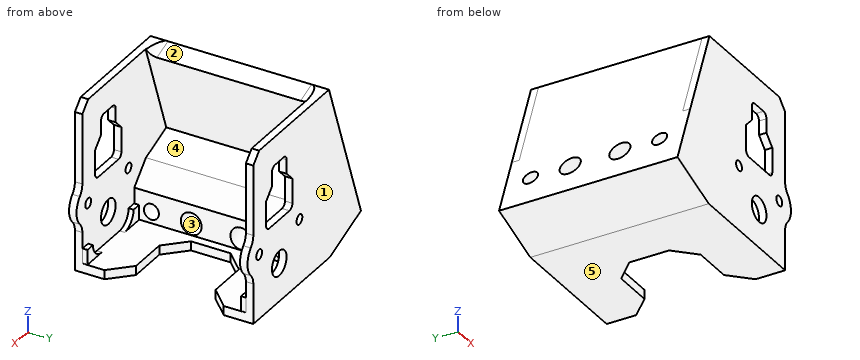
from build123d import *

# Parameters (mm, degrees)
SKETCH1_W                  = 17.8
SKETCH1_H                  = 30
SKETCH1_R                  = 1
SKETCH1_R_2                = 2.5
BOSS_EXTRUDE1_DEPTH        = 1.5
SKETCH2_W                  = 9
SKETCH2_H                  = 6
SKETCH2_W_2                = 5
SKETCH2_H_2                = 5.830943002
CUT_EXTRUDE1_DEPTH         = 20.247337478
CHAMFER1_SIZE              = 2
FILLET1_R                  = 1
BOSS_EXTRUDE2_DEPTH        = 1
SKETCH4_W                  = 12
SKETCH4_H                  = 17.95
BOSS_EXTRUDE3_DEPTH        = 4
BOSS_EXTRUDE4_DEPTH        = 35.9
SKETCH6_W                  = 12.770133269
SKETCH6_H                  = 35.9
BOSS_EXTRUDE5_DEPTH        = 11.41
F_3_0_MM_DOWEL_HOLES1_D    = 3
F_4_2_4_2_DIAMETER_HOLE1_D = 4.2
SKETCH12_W                 = 17.8
SKETCH12_H                 = 1.5
BOSS_EXTRUDE6_DEPTH        = 4
CHAMFER2_SIZE              = 2
SKETCH13_W                 = 26.167642811
SKETCH13_H                 = 35.9
BOSS_EXTRUDE7_DEPTH        = 1.840000002
CHAMFER3_SIZE              = 4
CHAMFER4_SIZE              = 4
SKETCH14_W                 = 16
SKETCH14_H                 = 8
CUT_EXTRUDE2_DEPTH         = 56.735892419
CHAMFER5_SIZE              = 4
BOSS_EXTRUDE8_DEPTH        = 1.5
BOSS_EXTRUDE9_START        = -34.4
BOSS_EXTRUDE9_DEPTH        = 1.5
FILLET2_R                  = 3
BOSS_EXTRUDE10_START       = -1.5
BOSS_EXTRUDE10_DEPTH       = 1.5
BOSS_EXTRUDE11_START       = -35.9
BOSS_EXTRUDE11_DEPTH       = 1.5
SKETCH18_W                 = 19.259010622
SKETCH18_H                 = 32.9
BOSS_EXTRUDE12_DEPTH       = 4
FILLET3_R                  = 2


# Some blends are built 0.0001 mm under size
with BuildPart() as part:
    # Sketch1 → Boss-Extrude1 (new body)
    with BuildSketch(Plane(origin=(0, 0, 0), x_dir=(1, 0, 0), z_dir=(0, 1, 0))):
        with Locations((0, -2)):
            Rectangle(SKETCH1_W, SKETCH1_H)
        with Locations(Location((-6.9, 0, 0), (0, 0, 270))):
            Circle(SKETCH1_R, mode=Mode.SUBTRACT)
        with Locations(Location((6.9, 0, 0), (0, 0, 270))):
            Circle(SKETCH1_R, mode=Mode.SUBTRACT)
        with Locations(Location((0, 5.3, 0), (0, 0, 270))):
            Circle(SKETCH1_R_2, mode=Mode.SUBTRACT)
    extrude(amount=BOSS_EXTRUDE1_DEPTH)

    # Sketch2 → Cut-Extrude1 (cut, through all)
    with BuildSketch(Plane(origin=(0, 1.5, 0), x_dir=(1, 0, 0), z_dir=(0, 1, 0))):
        with Locations((0, -6.5)):
            Rectangle(SKETCH2_W, SKETCH2_H)
        with Locations((0, -12.415471501)):
            Rectangle(SKETCH2_W_2, SKETCH2_H_2)
    extrude(amount=-CUT_EXTRUDE1_DEPTH, mode=Mode.SUBTRACT)

    # Chamfer1
    chamfer1_edges = [part.edges().sort_by_distance(p)[0] for p in [
        (2.5, 0.75, 9.5),
        (-2.5, 0.75, 9.5),
    ]]
    chamfer(chamfer1_edges, length=CHAMFER1_SIZE - 0.0001)  # a hair under: the kernel refuses the full size

    # Fillet1
    fillet1_edges = [part.edges().sort_by_distance(p)[0] for p in [
        (4.5, 0.75, 3.5),
        (2.5, 0.75, 15.330943002),
        (-2.5, 0.75, 15.330943002),
        (-4.5, 0.75, 3.5),
    ]]
    fillet(fillet1_edges, radius=FILLET1_R)

    # Sketch3 → Boss-Extrude2 (add)
    with BuildSketch(Plane(origin=(0, 1.5, 0), x_dir=(1, 0, 0), z_dir=(0, 1, 0))):
        with BuildLine():
            Line((8.84, 8.16), (6.959390471, 8.16))
            ThreePointArc((6.959390471, 8.16), (6.042112051, 10.284532913), (3.900010938, 11.159999998))
            Line((3.900010938, 11.159999998), (-3.900010938, 11.159999998))
            ThreePointArc((-3.900010938, 11.159999998), (-6.04211205, 10.284532912), (-6.959390471, 8.16))
            Line((-6.959390471, 8.16), (-8.84, 8.16))
            Line((-8.84, 8.16), (-8.84, 12.94))
            Line((-8.84, 12.94), (8.84, 12.94))
            Line((8.84, 12.94), (8.84, 8.16))
        make_face()
    extrude(amount=BOSS_EXTRUDE2_DEPTH)

    # Sketch4 → Boss-Extrude3 (add)
    with BuildSketch(Plane.ZY.offset(8.9)):
        with Locations((-7, 8.975)):
            Rectangle(SKETCH4_W, SKETCH4_H)
    extrude(amount=BOSS_EXTRUDE3_DEPTH)

    # Mirror2: part across plane


with BuildPart() as part_1:
    add(part.part)
    add(part.part.mirror(Plane.ZX.offset(17.95)))

    # Sketch5 → Boss-Extrude4 (add)
    with BuildSketch(Plane(origin=(0, 35.9, 0), x_dir=(1, 0, 0), z_dir=(0, 1, 0))):
        Polygon((-12.9, 1), (-17.267642811, 13), (-12.9, 13), align=None)
    extrude(amount=-BOSS_EXTRUDE4_DEPTH)

    # Sketch6 → Boss-Extrude5 (add)
    with BuildSketch(Plane(origin=(-11.069592853, 0, 4.029002304), x_dir=(0.3420201433256634, 0, 0.9396926207859103), z_dir=(-0.9396926207859103, 0, 0.3420201433256634))):
        with Locations((-11.736819105, 17.95)):
            Rectangle(SKETCH6_W, SKETCH6_H)
    extrude(amount=BOSS_EXTRUDE5_DEPTH)

    # Ø3.0 mm Dowel Holes1 (through all)
    with Locations(Plane(origin=(-23.72675034, 0, 2.614356121), x_dir=(-0.34202014332566333, 0, -0.9396926207859103), z_dir=(-0.9396926207859104, 0, 0.3420201433256634))):
        with Locations((5.693417073, -4.95), (5.693417073, -30.95)):
            Hole(F_3_0_MM_DOWEL_HOLES1_D / 2)

    # Ø4.2 (4.2) Diameter Hole1 (through all)
    with Locations(Plane(origin=(-21.791485656, 0, 7.931452139), x_dir=(0.34202014332566333, 0, 0.9396926207859103), z_dir=(-0.9396926207859104, 0, 0.3420201433256634))):
        with Locations((-11.35175247, 12.95), (-11.35175247, 22.95)):
            Hole(F_4_2_4_2_DIAMETER_HOLE1_D / 2)

    # Sketch12 → Boss-Extrude6 (add)
    with BuildSketch(Plane.XY.offset(17)):
        with Locations((0, 35.15)):
            Rectangle(SKETCH12_W, SKETCH12_H)
        with Locations((0, 0.75)):
            Rectangle(SKETCH12_W, SKETCH12_H)
    extrude(amount=BOSS_EXTRUDE6_DEPTH)

    # Chamfer2
    chamfer2_edges = [part_1.edges().sort_by_distance(p)[0] for p in [
        (8.9, 35.15, 21),
        (-8.9, 35.15, 21),
        (-8.9, 0.75, 21),
        (8.9, 0.75, 21),
    ]]
    chamfer(chamfer2_edges, length=CHAMFER2_SIZE)

    # Sketch13 → Boss-Extrude7 (add)
    with BuildSketch(Plane(origin=(0, 0, -13), x_dir=(-1, 0, 0), z_dir=(0, 0, -1))):
        with Locations((4.183821406, 17.95)):
            Rectangle(SKETCH13_W, SKETCH13_H)
    extrude(amount=-BOSS_EXTRUDE7_DEPTH)

    # Chamfer3
    # the kernel refuses this chamfer: 4 mm, written as the material it adds along each edge
    with BuildSketch(Plane(origin=(-8.9, 0, -1), x_dir=(-0.9996219169112968, 0, -0.027495876610586216), z_dir=(0, 1, 0)), Plane(origin=(-8.9, 35.9, -1), x_dir=(0.027495876610586924, 0, 0.9996219169112968), z_dir=(0, -1, 0))) as chamfer3_piece_1:
        Polygon((CHAMFER3_SIZE * 0.999621916911, CHAMFER3_SIZE * 0.0274958766106), (-CHAMFER3_SIZE * 0.0274958766106, CHAMFER3_SIZE * 0.999621916911), (0, 0), align=None)
    extrude(amount=1.5)

    # Chamfer4
    chamfer4_edges = [part_1.edges().sort_by_distance(p)[0] for p in [
        (-8.9, 17.95, -1),
    ]]
    chamfer(chamfer4_edges, length=CHAMFER4_SIZE - 0.0001)  # a hair under: the kernel refuses the full size

    # Sketch14 → Cut-Extrude2 (cut, through all)
    with BuildSketch(Plane.XY.offset(-11.159999998)):
        with Locations((0.9, 21.95)):
            Rectangle(SKETCH14_W, SKETCH14_H)
        with Locations((0.9, 13.95)):
            Rectangle(SKETCH14_W, SKETCH14_H)
    extrude(amount=-CUT_EXTRUDE2_DEPTH, mode=Mode.SUBTRACT)

    # Chamfer5
    chamfer5_edges = [part_1.edges().sort_by_distance(p)[0] for p in [
        (-7.1, 9.95, -12.079999999),
        (-7.1, 25.95, -12.079999999),
        (8.9, 25.95, -12.079999999),
        (8.9, 9.95, -12.079999999),
    ]]
    chamfer(chamfer5_edges, length=CHAMFER5_SIZE)

    # Sketch15 → Boss-Extrude8 (add)
    with BuildSketch(Plane.XZ):
        with BuildLine():
            Line((8.9, 3.464101615), (8.9, -3.464101615))
            ThreePointArc((8.9, -3.464101615), (10.9, 0), (8.9, 3.464101615))
        make_face()
    extrude(amount=-BOSS_EXTRUDE8_DEPTH)

    # Sketch15<2> → Boss-Extrude9 (add)
    with BuildSketch(Plane.XZ.offset(BOSS_EXTRUDE9_START)):
        with BuildLine():
            Line((8.9, 3.464101615), (8.9, -3.464101615))
            ThreePointArc((8.9, -3.464101615), (10.9, 0), (8.9, 3.464101615))
        make_face()
    extrude(amount=-BOSS_EXTRUDE9_DEPTH)

    # Fillet2
    fillet2_edges = [part_1.edges().sort_by_distance(p)[0] for p in [
        (-12.9, 0.75, -1),
        (-12.9, 35.15, -1),
        (-8.9, 0.75, 3),
        (-8.9, 35.15, 3),
        (8.9, 0.75, -3.464101615),
        (8.9, 0.75, 3.464101615),
        (8.9, 35.15, 3.464101615),
        (8.9, 35.15, -3.464101615),
    ]]
    fillet(fillet2_edges, radius=FILLET2_R)

    # Sketch16 → Boss-Extrude10 (add)
    with BuildSketch(Plane(origin=(0, 35.9, 0), x_dir=(1, 0, 0), z_dir=(0, 1, 0)).offset(BOSS_EXTRUDE10_START)):
        with BuildLine():
            Line((-8.9, -4.242640687), (-8.9, -19))
            Line((-8.9, -19), (-6.9, -21))
            Line((-6.9, -21), (-17.03492323, -21))
            Line((-17.03492323, -21), (-23.621892803, -2.902449835))
            Line((-23.621892803, -2.902449835), (-14.695950669, 0.346327414))
            ThreePointArc((-14.695950669, 0.346327414), (-13.020571397, 0.456137573), (-11.548569895, -0.351430105))
            Line((-11.548569895, -0.351430105), (-9.778679656, -2.121320344))
            ThreePointArc((-9.778679656, -2.121320344), (-9.128361402, -3.09459039), (-8.9, -4.242640687))
        make_face()
    extrude(amount=BOSS_EXTRUDE10_DEPTH)

    # Sketch16<2> → Boss-Extrude11 (add)
    with BuildSketch(Plane(origin=(0, 35.9, 0), x_dir=(1, 0, 0), z_dir=(0, 1, 0)).offset(BOSS_EXTRUDE11_START)):
        with BuildLine():
            Line((-8.9, -4.242640687), (-8.9, -19))
            Line((-8.9, -19), (-6.9, -21))
            Line((-6.9, -21), (-17.03492323, -21))
            Line((-17.03492323, -21), (-23.621892803, -2.902449835))
            Line((-23.621892803, -2.902449835), (-14.695950669, 0.346327414))
            ThreePointArc((-14.695950669, 0.346327414), (-13.020571397, 0.456137573), (-11.548569895, -0.351430105))
            Line((-11.548569895, -0.351430105), (-9.778679656, -2.121320344))
            ThreePointArc((-9.778679656, -2.121320344), (-9.128361402, -3.09459039), (-8.9, -4.242640687))
        make_face()
    extrude(amount=BOSS_EXTRUDE11_DEPTH)

    # Sketch18 → Boss-Extrude12 (add)
    with BuildSketch(Plane(origin=(-21.791485656, 0, 7.931452139), x_dir=(0.34202014332566333, 0, 0.9396926207859103), z_dir=(-0.9396926207859104, 0, 0.3420201433256634))):
        with Locations((4.277752841, 17.95)):
            Rectangle(SKETCH18_W, SKETCH18_H)
    extrude(amount=-BOSS_EXTRUDE12_DEPTH)

    # Fillet3
    # the kernel refuses this fillet: 2 mm, written as the material it adds along each edge
    with BuildSketch(Plane(origin=(-21.733386334, 34.4, 22.710100717), x_dir=(0.3420201433256634, 0, 0.9396926207859104), z_dir=(0.9396926207859104, 0, -0.3420201433256634))) as fillet3_piece_1_section:
        with BuildLine():
            CenterArc((FILLET3_R, FILLET3_R), FILLET3_R, 180, 90)
            Line((0, FILLET3_R), (0, 0))
            Line((0, 0), (FILLET3_R, 0))
        make_face()
    fillet3_piece_1 = extrude(amount=9, mode=Mode.PRIVATE)
    fillet3_piece_1 = split(fillet3_piece_1, bisect_by=Plane(origin=(-14.648893953, 33.872369462, 21), z_dir=(0, 0, -1)), keep=Keep.TOP, mode=Mode.PRIVATE)
    add(fillet3_piece_1)
    with BuildSketch(Plane(origin=(-21.733386334, 1.5, 22.710100717), x_dir=(0, 1, 0), z_dir=(0.9396926207859104, 0, -0.3420201433256634))) as fillet3_piece_2_section:
        with BuildLine():
            CenterArc((FILLET3_R, FILLET3_R), FILLET3_R, 180, 90)
            Line((0, FILLET3_R), (0, 0))
            Line((0, 0), (FILLET3_R, 0))
        make_face()
    fillet3_piece_2 = extrude(amount=9, mode=Mode.PRIVATE)
    fillet3_piece_2 = split(fillet3_piece_2, bisect_by=Plane(origin=(-14.648893954, 2.027630538, 21), z_dir=(0, 0, -1)), keep=Keep.TOP, mode=Mode.PRIVATE)
    add(fillet3_piece_2)


solid = part_1.part
Geometry check sheet. Reference: the model listing, model coordinates, mm. Face numbers are marked on the shaded views. A direction names the side the tool comes from. Give positions to 0.01 mm unless a question says otherwise; leave off trailing zeros.
1. Scan lines: line 1 (Y direction, x = -11, z = -1); line 2 (X direction, y = 34.95, z = 0); line 3 (Z direction, x = -1.5, y = 33.5). Record each from-to range of solid material in increasing order.
Completed:
line 1: y = 0 to 1.5, 34.4 to 35.9
line 2: x = -24.68 to -7.9, -5.9 to 5.9, 7.9 to 10.9
line 3: z = -13 to -11.16
2. Depth check by flat-ended pin: pin 1 (12 mm diameter, centred on y = 9.5, z = -2.5, fed in from -X); pin 2 (2 mm diameter, centred on x = -7, y = 4, fed in from +Z); pin 3 (6 mm diameter, centred on x = -18, y = 27.5, fed in from +Z). Enter the tip coordinate at first touch or a pass-through.
Completed:
pin 1: stops at x = -27.77
pin 2: stops at z = -11.16
pin 3: stops at z = 21
3. Draft check along Z on the marked faces 1, 2 and 3. Enter one of: pulls with the +Z half, pulls with the -Z half, needs draft (parallel to the pull), parting line crosses it, or undercut.
Completed:
face 1: needs draft
face 2: pulls with the +Z half
face 3: undercut
4. Sectioned sample at B-B (x = -11). State how many separate pieces and enclosed holes the cut face has, then the cut area to 3 significant figures.
Completed:
separate pieces: 1
enclosed holes: 4
area: 390 mm2
5. Access from +Z, -Z, +X, -X, +Y, -Y to the whole of each face (thin tool, end or side, straight path). Record for the marked faces 4 and 5.
Completed:
face 4: +X
face 5: -Z, +X, -X, +Y, -Y
